For this review, take the finished solid that the model builds, in its own axes (mm). A direction names the side the tool comes from. Round coordinates to 2 decimals unless told otherwise and drop trailing zeros. Order: outer loops, then holes, each group sorted by start corner. A loop starts at its lowest first (then second) coordinate and runs counter-clockwise, first axis right, second up. Notation, with made-up numbers: (-27, 8) -> (-10, 8) arc R12 ccw to (-10, 17) -> close; hole circle Ø2 at (47, -15.5). An arc over 180 degrees is marked (long way). Put each result on its own line as item: value. Start each with the question number.
```python
from build123d import *

# Parameters (mm, degrees)
SKETCH1_R               = 94.996
SKETCH1_R_2             = 53.975
TOP_OF_HATCH_DEPTH      = 3.302
SKETCH2_R               = 94.996
SKETCH2_R_2             = 89.789
HATCH_BODY_DEPTH        = 259.08
SKETCH3_R               = 13.335
CHARGE_TUBE_HOLES_DEPTH = 263.382
SKETCH4_R               = 3.81
BOLT_HOLES_DEPTH        = 263.382
SKETCH_5_R              = 5.08
ANTENNA_HOLES_DEPTH     = 263.382
SKETCH5_R               = 3.81
SKETCH5_R_2             = 3.175
INNER_SCREW_HOLES_DEPTH = 263.382
SKETCH8_R               = 1.397
CUT_EXTRUDE1_DEPTH      = 190.992
CUT_EXTRUDE3_DEPTH      = 263.3820001


with BuildPart() as part:
    # Sketch1 → Top of Hatch (new body)
    with BuildSketch(Plane(origin=(0, 0, 0), x_dir=(1, 0, 0), z_dir=(0, 1, 0))):
        Circle(SKETCH1_R)
        Circle(SKETCH1_R_2, mode=Mode.SUBTRACT)
    extrude(amount=TOP_OF_HATCH_DEPTH)

    # Sketch2 → Hatch Body (add)
    with BuildSketch(Plane(origin=(0, 3.302, 0), x_dir=(1, 0, 0), z_dir=(0, 1, 0))):
        Circle(SKETCH2_R)
        Circle(SKETCH2_R_2, mode=Mode.SUBTRACT)
    extrude(amount=HATCH_BODY_DEPTH)

    # Sketch3 → Charge Tube Holes (cut, through all)
    with BuildSketch(Plane.XZ):
        with Locations((-76.454, 0)):
            Circle(SKETCH3_R)
        with Locations((76.454, 0)):
            Circle(SKETCH3_R)
    extrude(amount=-CHARGE_TUBE_HOLES_DEPTH, mode=Mode.SUBTRACT)

    # Sketch4 → Bolt Holes (cut, through all)
    with BuildSketch(Plane.XZ):
        with Locations((-38.1, -65.991135768)):
            Circle(SKETCH4_R)
        with Locations((-38.1, 65.991135768)):
            Circle(SKETCH4_R)
        with Locations((38.1, 65.991135768)):
            Circle(SKETCH4_R)
        with Locations((38.1, -65.991135768)):
            Circle(SKETCH4_R)
    extrude(amount=-BOLT_HOLES_DEPTH, mode=Mode.SUBTRACT)

    # Sketch 5 → Antenna Holes (cut, through all)
    with BuildSketch(Plane.XZ):
        with Locations((-26.112352144, 57.324838678)):
            Circle(SKETCH_5_R)
        with Locations((9.193647856, 61.033450854)):
            Circle(SKETCH_5_R)
    extrude(amount=-ANTENNA_HOLES_DEPTH, mode=Mode.SUBTRACT)

    # Sketch5 → Inner Screw Holes (cut, through all)
    with BuildSketch(Plane.XZ):
        with Locations((58.42, 0)):
            Circle(SKETCH5_R)
        with Locations((-58.42, 0)):
            Circle(SKETCH5_R)
        with Locations((39.878, 41.91)):
            Circle(SKETCH5_R_2)
        with Locations((-39.878, 41.91)):
            Circle(SKETCH5_R_2)
        with Locations((39.878, -41.91)):
            Circle(SKETCH5_R_2)
        with Locations((-39.878, -41.91)):
            Circle(SKETCH5_R_2)
    extrude(amount=-INNER_SCREW_HOLES_DEPTH, mode=Mode.SUBTRACT)

    # Sketch8 → Cut-Extrude1 (cut, through all)
    with BuildSketch(Plane(origin=(94.996, 0, 0), x_dir=(0, 0, -1), z_dir=(1, 0, 0))):
        with Locations((14.351, 198.882)):
            Circle(SKETCH8_R)
        with Locations((-14.351, 198.882)):
            Circle(SKETCH8_R)
    extrude(amount=-CUT_EXTRUDE1_DEPTH, mode=Mode.SUBTRACT)

    # Sketch12 → Cut-Extrude3 (cut, through all)
    with BuildSketch(Plane.XZ):
        with BuildLine():
            Line((-94.996, 0), (94.996, 0))
            ThreePointArc((94.996, 0), (0, 94.996), (-94.996, 0))
        make_face()
    extrude(amount=-CUT_EXTRUDE3_DEPTH, mode=Mode.SUBTRACT)


solid = part.part
```
Item 1: Consider section B-B, the plane y = 227.5. Write out the cut boundary in (x, z).
Item 2: Mouldability with a two-part tool opening along Z and no side actions: class faces 1 (the face through (-1, 0, -59)), 2 (the face through (-42.218, 1.628, -39.764)), 3 (the face through (1.974, 131.028, -89.767)) as +Z half, -Z half, draft (parallel to the pull), parting line (faces both ways), or undercut.
Item 3: For L1, parallel to Y at x = -55, z = -8; L2, parallel to X at y = 47, z = -50.5; L3, parallel to X at y = 55, z = -21, list the stretches that pass through material, from the lowest coordinate up.
Item 4: Consider section A-A, the plane z = -8. Write out the cut boundary in (x, y).
Item 5: Consider section C-C, the plane x = 0. Write out the cut boundary in (y, z) (3 decimals), plus the area to 3 significant figures.
Item 6: Consider section D-D, the plane z = -79. Write out the cut boundary in (x, y).
Item 7: Tool access review of faces 4 (the face through (76.16, 1.63, -13.33)), 5 (the face through (-1, 3.302, -55)): name each direction out of +Z, -Z, +X, -X, +Y, -Y from which nothing blocks a thin tool from reaching the whole face with its end or side.
Item 8: Insertion check: pin 1 Ø2.5 at (y, z) = (198.882, -14.351) entering from +X; pin 2 Ø6 at (x, y) = (1.5, 42.5) entering from +Z; pin 3 Ø6 at (y, z) = (124.5, -62.5) entering from +X; pin 4 Ø2 at (x, y) = (51.5, 151.5) entering from -Z. Each pin has a flat end and moves straight along its axis. Give the tip position at first contact, or say it passes through.
Evaluation:
1. outline: (-95, 0) arc R95 ccw to (95, 0) -> (89.79, 0) arc R89.79 cw to (-89.79, 0) -> close
2. face 1: draft
2. face 2: undercut
2. face 3: +Z half
3. L1: y = 0 to 3.3
3. L2: x = -80.46 to -74.24, 74.24 to 80.46
3. L3: x = -92.65 to -87.3, 87.3 to 92.65
4. outline: (-94.66, 0) -> (-87.12, 0) -> (-87.12, 3.3) -> (-89.43, 3.3) -> (-89.43, 262.38) -> (-94.66, 262.38) -> close; (-65.79, 0) -> (-53.38, 0) -> (-53.38, 3.3) -> (-65.79, 3.3) -> close; (53.38, 0) -> (65.79, 0) -> (65.79, 3.3) -> (53.38, 3.3) -> close; (87.12, 0) -> (94.66, 0) -> (94.66, 262.38) -> (89.43, 262.38) -> (89.43, 3.3) -> (87.12, 3.3) -> close
5. outline: (0, -94.996) -> (262.382, -94.996) -> (262.382, -89.789) -> (3.302, -89.789) -> (3.302, -53.975) -> (0, -53.975) -> close
5. area: 1,480 mm^2
6. outline: (-52.76, 0) -> (52.76, 0) -> (52.76, 262.38) -> (42.67, 262.38) -> (42.67, 3.3) -> (-42.67, 3.3) -> (-42.67, 262.38) -> (-52.76, 262.38) -> close
7. face 4: +Z, +Y, -Y
7. face 5: +Z, +Y
8. pin 1: passes through
8. pin 2: stops at z = -89.68
8. pin 3: stops at x = 74.05
8. pin 4: stops at z = -80.46
